Geometry check sheet. Reference: the model listing, model coordinates, mm. A direction names the side the tool comes from. Coordinates: 2 decimals unless noted, no trailing zeros. Loops run counter-clockwise (first coordinate to the right, second up) from the corner with the lowest first, then second, coordinate; pieces in that order, holes last.
from build123d import *

# Parameters (mm, degrees)
SKETCH1_W           = 7.985890062
SKETCH1_H           = 3.00014889
SKETCH1_W_2         = 7.985890063
SKETCH1_H_2         = 3.000080527
BOSS_EXTRUDE1_DEPTH = 3.175


with BuildPart() as part:
    # Sketch1 → Boss-Extrude1 (new body)
    with BuildSketch(Plane(origin=(0, 0, 0), x_dir=(1, 0, 0), z_dir=(0, 1, 0))):
        with BuildLine():
            Line((8.450778283, -13.38162857), (8.406948402, -13.382009456))
            Line((8.406948402, -13.382009456), (5.43267765, -13.382009456))
            Line((5.43267765, -13.382009456), (5.476497782, -13.38162857))
            Line((5.476497782, -13.38162857), (5.476497782, -7.251478059))
            Line((5.476497782, -7.251478059), (1.483591746, -7.251478059))
            Line((1.483591746, -7.251478059), (1.483591746, -8.50154498))
            Line((1.483591746, -8.50154498), (-1.012030582, -8.50154498))
            Line((-1.012030582, -8.50154498), (-1.012030582, -7.251478059))
            Line((-1.012030582, -7.251478059), (-3.507584669, -7.251478059))
            Line((-3.507584669, -7.251478059), (-3.507584669, -4.251397533))
            Line((-3.507584669, -4.251397533), (-1.012030582, -4.251397533))
            Line((-1.012030582, -4.251397533), (-1.012030582, -3.001320846))
            Line((-1.012030582, -3.001320846), (1.483591746, -3.001320846))
            Line((1.483591746, -3.001320846), (1.483591746, -4.251397533))
            Line((1.483591746, -4.251397533), (5.476497782, -4.251397533))
            Line((5.476497782, -4.251397533), (5.476497782, 20.246361134))
            Line((5.476497782, 20.246361134), (8.471221179, 20.246361134))
            Line((8.471221179, 20.246361134), (8.471221179, 28.246728876))
            Line((8.471221179, 28.246728876), (-16.804601477, 28.246728876))
            Line((-16.804601477, 28.246728876), (-16.804601477, 23.246510025))
            Line((-16.804601477, 23.246510025), (-13.809887829, 23.246510025))
            Line((-13.809887829, 23.246510025), (-13.809887829, 7.746043514))
            Line((-13.809887829, 7.746043514), (-9.816981793, 7.746043514))
            Line((-9.816981793, 7.746043514), (-9.816981793, 8.996110434))
            Line((-9.816981793, 8.996110434), (-7.321417957, 8.996110434))
            Line((-7.321417957, 8.996110434), (-7.321417957, 7.746043514))
            Line((-7.321417957, 7.746043514), (-4.825805378, 7.746043514))
            Line((-4.825805378, 7.746043514), (-4.825805378, 4.745894623))
            Line((-4.825805378, 4.745894623), (-7.321417957, 4.745894623))
            Line((-7.321417957, 4.745894623), (-7.321417957, 3.495827702))
            Line((-7.321417957, 3.495827702), (-9.816981793, 3.495827702))
            Line((-9.816981793, 3.495827702), (-9.816981793, 4.745894623))
            Line((-9.816981793, 4.745894623), (-13.809887829, 4.745894623))
            Line((-13.809887829, 4.745894623), (-13.809887829, -24.255271193))
            Line((-13.809887829, -24.255271193), (-16.804601477, -24.255271193))
            Line((-16.804601477, -24.255271193), (-16.804601477, -31.755565288))
            Line((-16.804601477, -31.755565288), (0.529541194, -31.755565288))
            Line((0.529541194, -31.755565288), (0.529541194, -25.875998513))
            add(Edge.make_bspline(
                [(0.529541194, -25.875998513), (0.529541194, -24.216108328), (1.884173069, -23.980760021), (3.543615638, -23.915862955)],
                knots=[38, 38, 38, 38, 39, 39, 39, 39], degree=3))
            add(Edge.make_bspline(
                [(3.543615638, -23.915862955), (5.651300627, -23.833288885), (5.482317719, -23.277547326), (5.43267765, -18.755056825)],
                knots=[39, 39, 39, 39, 40, 40, 40, 40], degree=3))
            add(Edge.make_bspline(
                [(5.43267765, -18.755056825), (6.324629372, -18.755056826), (7.369010812, -18.755056826), (8.450778283, -18.755056826)],
                knots=[40, 40, 40, 40, 41, 41, 41, 41], degree=3))
            Line((8.450778283, -18.755056826), (8.450778283, -13.38162857))
        make_face()
        with Locations((-4.805196753, 18.048513823)):
            Rectangle(SKETCH1_W, SKETCH1_H, mode=Mode.SUBTRACT)
        with Locations((-4.805196754, -15.272154822)):
            Rectangle(SKETCH1_W_2, SKETCH1_H_2, mode=Mode.SUBTRACT)
    extrude(amount=BOSS_EXTRUDE1_DEPTH)


solid = part.part
(1) Draft check along X on faces 1 (the flat face through (-16.805, 2, -26)), 2 (the flat face through (-4, 3.175, 1)), 3 (the flat face through (-0.812, 2, 15)), 4 (the flat face through (-1.012, 2, 8)). Enter one of: +X half, -X half, draft (parallel to the pull), parting line (faces both ways), or undercut.
Findings:
face 1: -X half
face 2: draft
face 3: undercut
face 4: undercut
(2) Gauge pin test, flat ends, axial feed: pin 1 Ø1 at (y, z) = (2.5, 6) entering from -X; pin 2 Ø0.6 at (y, z) = (1, -4.5) entering from +X. Record the tip position at first contact, or that the pin passes through.
Findings:
pin 1: stops at x = -13.81
pin 2: stops at x = 5.48
(3) Access from +Z, -Z, +X, -X, +Y, -Y to the whole of each face (thin tool, end or side, straight path). Record for faces 5 (the flat face through (-2, 2, 7.251)), 6 (the flat face through (-4.826, 2, -6)), 7 (the flat face through (-5, 2, 13.772)).
Findings:
face 5: +X, +Y, -Y
face 6: -X, +Y, -Y
face 7: +Y, -Y
(4) Sectioned sample at A-A on z = -10. Record the cut outline in (x, y) (1 decimal).
Findings:
outline: (-13.8, 0) - (5.5, 0) - (5.5, 3.2) - (-13.8, 3.2) - close
(5) Sectioned sample at B-B on y = 2.45. State how many separate pieces and enclosed holes the cut face has, and give its area (3 significant figures).
Findings:
separate pieces: 1
enclosed holes: 2
area: 1,080 mm2
(6) Sectioned sample at C-C on z = 5. Record the cut outline in (x, y) (3 decimals).
Findings:
outline: (-13.81, 0) - (-3.508, 0) - (-3.508, 3.175) - (-13.81, 3.175) - close
(7) Scan lines: L1, parallel to Z at x = -1.75, y = 0.5; L2, parallel to Z at x = -4.75, y = 0.65; L3, parallel to Z at x = 6.75, y = 2.2. Record each from-to range of solid material in increasing order.
Findings:
L1: z = -28.25 to -19.55, -16.55 to 4.25, 7.25 to 13.77, 16.77 to 31.76
L2: z = -28.25 to -19.55, -16.55 to 13.77, 16.77 to 31.76
L3: z = -28.25 to -20.25, 13.38 to 18.76
